Can you work these out from the model? Positions are in its coordinate system, mm. A direction names the side the tool comes from. Give positions to 0.01 mm unless a question says otherwise; leave off trailing zeros. Write each loop counter-clockwise with the first axis right and the second up, starting at its lowest first coordinate (ties: lowest second). Pieces come first, ordered by that corner, then holes. Notation, with made-up numbers: (-27, -32) - (-23, -32) arc R32 cw to (-23, -4) - close; hole circle Ø7 at (-26.5, -22.5). An arc over 180 degrees is marked (long way). Use a Markdown table: item, result. Add a question column.
```python
from build123d import *

# Parameters (mm, degrees)
SKETCH1_W          = 100
SKETCH1_H          = 7
BASE_EXTRUDE_DEPTH = 25
CUT_EXTRUDE1_DEPTH = 8
SKETCH3_R          = 2.5
CUT_EXTRUDE2_DEPTH = 8


with BuildPart() as part:
    # Sketch1 → Base-Extrude (new body)
    with BuildSketch(Plane.XY):
        with Locations((50, 3.5)):
            Rectangle(SKETCH1_W, SKETCH1_H)
    extrude(amount=BASE_EXTRUDE_DEPTH)

    # Sketch2 → Cut-Extrude1 (cut, through all)
    with BuildSketch(Plane(origin=(0, 7, 0), x_dir=(-1, 0, 0), z_dir=(0, 1, 0))):
        with BuildLine():
            Line((-94, 9.5), (-94, 15.5))
            ThreePointArc((-94, 15.5), (-85, 12.5), (-94, 9.5))
        make_face()
    extrude(amount=-CUT_EXTRUDE1_DEPTH, mode=Mode.SUBTRACT)

    # Sketch3 → Cut-Extrude2 (cut, through all)
    with BuildSketch(Plane(origin=(0, 7, 0), x_dir=(-1, 0, 0), z_dir=(0, 1, 0))):
        with Locations((-10, 12.5)):
            Circle(SKETCH3_R)
    extrude(amount=-CUT_EXTRUDE2_DEPTH, mode=Mode.SUBTRACT)


solid = part.part
```
Q1. On a 3-axis mill with a long thin cutter (end or side, diameter ignored), from which of +Z, -Z, +X, -X, +Y, -Y can I reach the whole of each face in a straight line? I mean faces 1 (the flat face through (94, 4, 12)), 2 (the flat face through (49, 7, 12)). Say none if no direction works.
Q2. Suppose I cut it at C-C (y = 2.5). Please give me the cut outline in (x, z), and give its area (3 significant figures).
Q3. If we mould it in two halves opening along X, with no side actions, what happens to faces 3 (the flat face through (49, 4, 25)), 4 (the cylindrical face through (85.003, 3.549, 12.675)), 5 (the flat face through (0, 3, 12)), 6 (the flat face through (100, 3, 12))? For each: released by +X, released by -X, zero draft, split by the parting line, or undercut.
Q4. I'm going to push a flat-ended pin straight in: P1, Ø3, axis at x = 10, z = 12.5, coming from the +Y side. Where does the tip first touch, or does it pass through?
Q5. If I drill on probe 1 along Z at (x, y) = (10, 4.5); probe 2 along Z at (x, y) = (90, 3.25); probe 3 along X at (y, z) = (4.5, 15.5), over which ranges is the centre line in solid material (lowest first)? Write a range as [from, to].
Q6. Suppose I cut it at B-B (x = 10). Please give me the cut outline in (y, z), and give its area (3 significant figures).
Q7. Suppose I cut it at A-A (z = 12.5). Please give me the cut outline in (x, y), and give its area (3 significant figures).
Q8. Suppose I cut it at D-D (x = 90). Please give me the cut outline in (y, z), and give its area (3 significant figures).
Derived:
| question | item | result |
|---|---|---|
| 1 | face 1 | +Y, -Y |
| 1 | face 2 | +Z, -Z, +X, -X, +Y |
| 2 | outline | (0, 0) - (100, 0) - (100, 25) - (0, 25) - close; hole circle Ø5 at (10, 12.5); hole (94, 9.5) - (94, 15.5) arc R5 ccw (long way) to start |
| 2 | area | 2,410 mm² |
| 3 | face 3 | zero draft |
| 3 | face 4 | undercut |
| 3 | face 5 | released by -X |
| 3 | face 6 | released by +X |
| 4 | P1 | through |
| 5 | probe 1 | [0, 10], [15, 25] |
| 5 | probe 2 | [0, 7.5], [17.5, 25] |
| 5 | probe 3 | [0, 86], [94, 100] |
| 6 | outline | (0, 0) - (7, 0) - (7, 10) - (0, 10) - close; (0, 15) - (7, 15) - (7, 25) - (0, 25) - close |
| 6 | area | 140 mm² |
| 7 | outline | (0, 0) - (7.5, 0) - (7.5, 7) - (0, 7) - close; (12.5, 0) - (85, 0) - (85, 7) - (12.5, 7) - close; (94, 0) - (100, 0) - (100, 7) - (94, 7) - close |
| 7 | area | 602 mm² |
| 8 | outline | (0, 0) - (7, 0) - (7, 7.5) - (0, 7.5) - close; (0, 17.5) - (7, 17.5) - (7, 25) - (0, 25) - close |
| 8 | area | 105 mm² |
